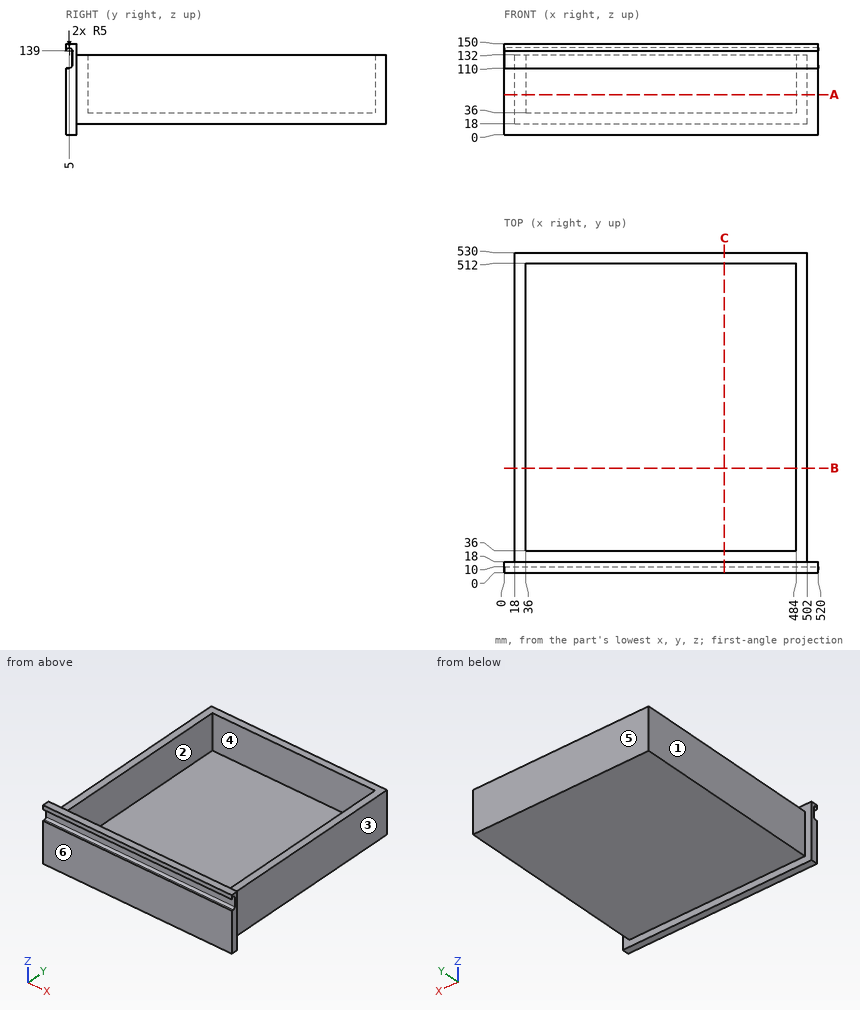
Can you work these out from the drawing? Everything is in mm from the part's minimum corner. A direction names the side the tool comes from. Round coordinates to 2 decimals unless told otherwise and drop trailing zeros. Loops run counter-clockwise (first coordinate to the right, second up) from the corner with the lowest first, then second, coordinate; pieces in that order, holes last. Notation, with made-up numbers: (-9.5, -25.75) - (9.5, -25.75) arc R21 ccw to (9.5, -6.75) - close; hole circle Ø4 at (60, -17.75). An arc over 180 degrees is marked (long way). Answer in a Markdown table with one row per item. Add a question column.
(1) If we section it at A-A (z = 66): Please give me the cut outline in (x, y), plus the area to 3 significant figures.
(2) If we mould it in two halves opening along Y, with no side actions, what happens to the marked faces 4, 5 and 6? For each: pulls with the +Y half, pulls with the -Y half, needs draft (parallel to the pull), parting line crosses it, or undercut.
(3) I'm going to push flat-ended pins straight in: pin 1 (3 mm diameter, centred on x = 282.5, z = 120.5, fed in from -Y); pin 2 (10 mm diameter, centred on x = 265.5, y = 321.5, fed in from -Z); pin 3 (1 mm diameter, centred on x = 52.5, y = 192.5, fed in from +Z). Where does each tip first touch, or does it pass through?
(4) For the marked faces 1, 2 and 3, which set-ups out of +Z, -Z, +X, -X, +Y, -Y let a thin tool reach every point of the face, with its end or its side?
(5) If we section it at B-B (y = 173): Please give me the cut outline in (x, z), plus the area to 3 significant figures.
(6) If we section it at C-C (x = 365): Please give me the cut outline in (y, z), plus the area to 3 significant figures.
(7) I need wall thicknesses on line 1 along X through (y, z) = (53.5, 74.5); line 2 along Y through (x, z) = (134.5, 83); line 3 along Y through (x, z) = (307.5, 126). Which ranges of each line are inside material? Lowest first, please.
Model answer:
| question | item | result |
|---|---|---|
| 1 | outline | (0, 0) - (520, 0) - (520, 18) - (502, 18) - (502, 530) - (18, 530) - (18, 18) - (0, 18) - close; hole (36, 36) - (484, 36) - (484, 512) - (36, 512) - close |
| 1 | area | 43,900 mm² |
| 2 | face 4 | undercut |
| 2 | face 5 | pulls with the +Y half |
| 2 | face 6 | pulls with the -Y half |
| 3 | pin 1 | stops at y = 10 |
| 3 | pin 2 | stops at z = 18 |
| 3 | pin 3 | stops at z = 36 |
| 4 | face 1 | +Z, -Z, -X, +Y |
| 4 | face 2 | +Z |
| 4 | face 3 | +Z, -Z, +X, +Y |
| 5 | outline | (18, 18) - (502, 18) - (502, 132) - (484, 132) - (484, 36) - (36, 36) - (36, 132) - (18, 132) - close |
| 5 | area | 12,200 mm² |
| 6 | outline | (0, 0) - (18, 0) - (18, 18) - (530, 18) - (530, 132) - (512, 132) - (512, 36) - (36, 36) - (36, 132) - (18, 132) - (18, 150) - (0, 150) - (0, 139) arc R5 cw to (10, 139) - (10, 115) arc R5 cw to (5, 110) - (0, 110) - close |
| 6 | area | 15,000 mm² |
| 7 | line 1 | x = 18 to 36, 484 to 502 |
| 7 | line 2 | y = 0 to 36, 512 to 530 |
| 7 | line 3 | y = 10 to 36, 512 to 530 |
